from build123d import *
from build123d.topology import SkipClean

# Parameters (mm, degrees)
EXTRUDE_1_DEPTH          = 42
EXTRUDE_3_DEPTH          = 3
EXTRUDE_3_DEPTH_BACK     = 45
SKETCH_2_R               = 15
SKETCH_2_R_2             = 9
CUT_EXTRUDE_1_DEPTH      = 78.136243103
CUT_EXTRUDE_1_DEPTH_BACK = 78.136243103
SKETCH_3_R               = 4
CUT_EXTRUDE_2_DEPTH      = 78.136243103
CUT_EXTRUDE_2_DEPTH_BACK = 78.136243103
SKETCH_4_R               = 4
FILLET_5_R               = 10


with BuildPart() as part:
    # Sketch 1 → Extrude 1 (new body)
    with BuildSketch(Plane.XY):
        with BuildLine():
            ThreePointArc((25, 15), (29.393398282, 4.393398282), (40, 0))
            ThreePointArc((40, 0), (50.606601718, 4.393398282), (55, 15))
            Line((55, 15), (49, 15))
            ThreePointArc((49, 15), (40, 6), (31, 15))
            Line((31, 15), (25, 15))
        make_face()
        with BuildLine():
            Line((49, 15), (55, 15))
            ThreePointArc((55, 15), (50.606601718, 25.606601718), (40, 30))
            ThreePointArc((40, 30), (29.393398282, 25.606601718), (25, 15))
            Line((25, 15), (31, 15))
            ThreePointArc((31, 15), (40, 24), (49, 15))
        make_face()
        with BuildLine():
            Line((20, 15), (25, 15))
            ThreePointArc((25, 15), (29.393398282, 25.606601718), (40, 30))
            Line((40, 30), (0, 30))
            Line((0, 30), (0, 21))
            Line((0, 21), (20, 21))
            Line((20, 21), (20, 15))
        make_face()
        with BuildLine():
            ThreePointArc((25, 15), (29.393398282, 4.393398282), (40, 0))
            ThreePointArc((40, 0), (50.606601718, 4.393398282), (55, 15))
            Line((55, 15), (49, 15))
            ThreePointArc((49, 15), (40, 6), (31, 15))
            Line((31, 15), (25, 15))
        make_face()
        with BuildLine():
            Line((49, 15), (55, 15))
            ThreePointArc((55, 15), (50.606601718, 25.606601718), (40, 30))
            ThreePointArc((40, 30), (29.393398282, 25.606601718), (25, 15))
            Line((25, 15), (31, 15))
            ThreePointArc((31, 15), (40, 24), (49, 15))
        make_face()
        with BuildLine():
            Line((0, 9), (0, 0))
            Line((0, 0), (40, 0))
            ThreePointArc((40, 0), (29.393398282, 4.393398282), (25, 15))
            Line((25, 15), (20, 15))
            Line((20, 15), (20, 9))
            Line((20, 9), (0, 9))
        make_face()
    extrude(amount=EXTRUDE_1_DEPTH)

    # Sketch 2 → Extrude 3 (add, two sides: drawn at the far end of the back side and taken through both)
    with SkipClean():  # the faces are left unmerged after this step: merging them gives an invalid solid
        with BuildSketch(Plane.XY.offset(42).offset(-EXTRUDE_3_DEPTH_BACK)):
            with Locations((40, 15)):
                Circle(SKETCH_2_R)
            with Locations(Location((40, 15, 0), (0, 0, 180))):
                Circle(SKETCH_2_R_2, mode=Mode.SUBTRACT)
        extrude(amount=EXTRUDE_3_DEPTH + EXTRUDE_3_DEPTH_BACK)
    add(part.part.scale(1), mode=Mode.REPLACE)  # the faces are merged on a copy

    # Sketch 3 → Cut-Extrude 1 (cut, two sides: drawn at the far end of the back side and taken through both)
    with SkipClean():  # the faces are left unmerged after this step: merging them gives an invalid solid
        with BuildSketch(Plane(origin=(0, 30, 0), x_dir=(1, 0, 0), z_dir=(0, 1, 0)).offset(-CUT_EXTRUDE_1_DEPTH_BACK)):
            with Locations(Location((10, -10, 0), (0, 0, 270))):
                Circle(SKETCH_3_R)
        extrude(amount=CUT_EXTRUDE_1_DEPTH + CUT_EXTRUDE_1_DEPTH_BACK, mode=Mode.SUBTRACT)

    # Sketch 4 → Cut-Extrude 2 (cut, two sides: drawn at the far end of the back side and taken through both)
    with SkipClean():  # the faces are left unmerged after this step: merging them gives an invalid solid
        with BuildSketch(Plane(origin=(0, 30, 0), x_dir=(1, 0, 0), z_dir=(0, 1, 0)).offset(-CUT_EXTRUDE_2_DEPTH_BACK)):
            with Locations(Location((10, -32, 0), (0, 0, 270))):
                Circle(SKETCH_4_R)
        extrude(amount=CUT_EXTRUDE_2_DEPTH + CUT_EXTRUDE_2_DEPTH_BACK, mode=Mode.SUBTRACT)

    # Fillet 5
    fillet_5_edges = [part.edges().sort_by_distance(p)[0] for p in [
        (0, 4.5, 42),
        (0, 4.5, 0),
        (0, 25.5, 0),
        (0, 25.5, 42),
    ]]
    fillet(fillet_5_edges, radius=FILLET_5_R)


solid = part.part
Read the model definition and answer for the solid it produces. Units are mm, in the model's axes. A direction names the side the tool comes from. Give positions to 0.01 mm unless a question says otherwise; leave off trailing zeros. Loops run counter-clockwise (first coordinate to the right, second up) from the corner with the lowest first, then second, coordinate; pieces in that order, holes last. Notation, with made-up numbers: (18, -14.75) - (64, -14.75) arc R12 cw to (64, -1.75) - close; hole circle Ø2 at (64, 72). An arc over 180 degrees is marked (long way). Answer as CSV lines item,"result". Start each with the question number.
1) Find section C-C (x = 16.5). Write down the section's boundary in (y, z).
2) Straight lines are drawn through the part: L1, parallel to Z at x = 10, y = 25.5; L2, parallel to Y at x = 15.5, z = 23; L3, parallel to Y at x = 40, z = -2.1. For each, find the intervals that lie inside material, in ascending order. Write a range as from..to.
3) Each of these flat-tipped pins is pushed along its axis until it touches: pin 1 Ø6 at (y, z) = (17, 15) entering from -X; pin 2 Ø2 at (y, z) = (21, 23.5) entering from +X; pin 3 Ø5 at (x, z) = (48.5, 37.5) entering from -Y. Where does it stop, or does it pass through?
4) Which of the six approach directions +Z, -Z, +X, -X, +Y, -Y give full straight-line access (tool end or side, diameter ignored) to faces 4 (the face through (10, 9, 21)), 5 (the face through (46.5, 8.5, -3))?
5) Find section A-A (z = 24.5). Write down the section's boundary in (x, y), then the cut area to 3 significant figures.
6) Determine the mould class of faces 1 (the face through (20, 15, 21)), 2 (the face through (10, 21, 21)), 3 (the face through (10, 25, 6)) for opening direction X: released by +X, released by -X, zero draft, split by the parting line, or undercut.
7) Find section B-B (z = 12). Write down the section's boundary in (x, y).
Findings below:
1,outline,"(0, 0) - (9, 0) - (9, 42) - (0, 42) - close; (21, 0) - (30, 0) - (30, 42) - (21, 42) - close"
2,L1,"0..6, 14..28, 36..42"
2,L2,"0..9, 21..30"
2,L3,"0..6, 24..30"
3,pin 1,"x = 20"
3,pin 2,"x = 54.14"
3,pin 3,"y = 1.25"
4,face 4,"+Z, -Z, -X"
4,face 5,"-Z, +X, -X, +Y, -Y"
5,outline,"(0, 0) - (40, 0) arc R15 ccw to (40, 30) - (0, 30) - (0, 21) - (20, 21) - (20, 9) - (0, 9) - close; hole circle Ø18 at (40, 15)"
5,area,"1,060 mm^2"
6,face 1,"released by -X"
6,face 2,"zero draft"
6,face 3,"undercut"
7,outline,"(0, 0) - (6.54, 0) - (6.54, 9) - (0, 9) - close; (0, 21) - (6.54, 21) - (6.54, 30) - (0, 30) - close; (13.46, 0) - (40, 0) arc R15 ccw to (40, 30) - (13.46, 30) - (13.46, 21) - (20, 21) - (20, 9) - (13.46, 9) - close; hole circle Ø18 at (40, 15)"
